Read the model definition and answer for the solid it produces. Units are mm, in the model's axes. A direction names the side the tool comes from. Coordinates: 2 decimals unless noted, no trailing zeros. Order: outer loops, then holes, each group sorted by start corner. A loop starts at its lowest first (then second) coordinate and runs counter-clockwise, first axis right, second up. Notation, with made-up numbers: M 83,-4 L 108,-4 A26 cw 108,28 Z; hole C -29.75,1.25 d9. An arc over 180 degrees is marked long. Put each result on its own line as item: value.
from build123d import *

# Parameters (mm, degrees)
BOSS_EXTRUDE1_DEPTH = 2.7
BOSS_EXTRUDE2_DEPTH = 0.6
FILLET1_R           = 0.5
FILLET2_R           = 2.5
FILLET3_R           = 0.5
FILLET4_R           = 1
SKETCH3_R           = 1
CUT_EXTRUDE1_DEPTH  = 15.611382549


with BuildPart() as part:
    # Sketch1 → Boss-Extrude1 (new body)
    with BuildSketch(Plane.XY):
        with BuildLine():
            Line((-1.082531755, 12.625), (-2.5, 10.169872981))
            Line((-2.5, 10.169872981), (-2.5, 2.449489743))
            ThreePointArc((-2.5, 2.449489743), (-3.463668402, -0.502992247), (-1.7, -3.059411708))
            Line((-1.7, -3.059411708), (-1.7, -7))
            Line((-1.7, -7), (-0.5, -7))
            Line((-0.5, -7), (-0.5, -1.414213562))
            ThreePointArc((-0.5, -1.414213562), (0, 1.5), (0.5, -1.414213562))
            Line((0.5, -1.414213562), (0.5, -7))
            Line((0.5, -7), (1.7, -7))
            Line((1.7, -7), (1.7, -3.059411708))
            ThreePointArc((1.7, -3.059411708), (3.388062941, 0.878082861), (0, 3.5))
            Line((0, 3.5), (0, 9.5))
            Line((0, 9.5), (1.082531755, 11.375))
            ThreePointArc((1.082531755, 11.375), (0.625, 13.082531755), (-1.082531755, 12.625))
        make_face()
    extrude(amount=BOSS_EXTRUDE1_DEPTH)

    # Sketch2 → Boss-Extrude2 (add)
    with BuildSketch(Plane.XY.offset(2.7)):
        with BuildLine():
            Line((0.5, -0.748331477), (0.5, -7))
            Line((0.5, -7), (1.7, -7))
            Line((1.7, -7), (1.7, -3.059411708))
            ThreePointArc((1.7, -3.059411708), (3.388062941, 0.878082861), (0, 3.5))
            Line((0, 3.5), (0, 9.5))
            Line((0, 9.5), (1.082531755, 11.375))
            ThreePointArc((1.082531755, 11.375), (0.625, 13.082531755), (-1.082531755, 12.625))
            Line((-1.082531755, 12.625), (-2.5, 10.169872981))
            Line((-2.5, 10.169872981), (-2.5, 2.449489743))
            ThreePointArc((-2.5, 2.449489743), (-3.463668402, -0.502992247), (-1.7, -3.059411708))
            Line((-1.7, -3.059411708), (-1.7, -7))
            Line((-1.7, -7), (-0.5, -7))
            Line((-0.5, -7), (-0.5, -0.748331477))
            ThreePointArc((-0.5, -0.748331477), (0, 0.9), (0.5, -0.748331477))
        make_face()
    extrude(amount=BOSS_EXTRUDE2_DEPTH)

    # Fillet1
    fillet1_edges = [part.edges().sort_by_distance(p)[0] for p in [
        (-0.5, -0.748331477, 3),
        (0.5, -0.748331477, 3),
    ]]
    fillet(fillet1_edges, radius=FILLET1_R)

    # Fillet2
    fillet2_edges = [part.edges().sort_by_distance(p)[0] for p in [
        (-2.5, 2.449489743, 1.65),
        (-2.5, 10.169872981, 1.65),
        (0, 9.5, 1.65),
        (0, 3.5, 1.65),
    ]]
    fillet(fillet2_edges, radius=FILLET2_R)

    # Fillet3
    fillet3_edges = [part.edges().sort_by_distance(p)[0] for p in [
        (-1.7, -3.059411708, 1.65),
        (1.7, -3.059411708, 1.65),
    ]]
    fillet(fillet3_edges, radius=FILLET3_R)

    # Fillet4
    fillet4_edges = [part.edges().sort_by_distance(p)[0] for p in [
        (-1.1, -7, 0),
        (1.1, -7, 0),
        (1.1, -7, 3.3),
        (-1.1, -7, 3.3),
    ]]
    fillet(fillet4_edges, radius=FILLET4_R)

    # Sketch3 → Cut-Extrude1 (cut, through all)
    with BuildSketch(Plane.ZY.offset(1.7)):
        with Locations((1.65, -5.170329309)):
            Circle(SKETCH3_R)
    extrude(amount=-CUT_EXTRUDE1_DEPTH, mode=Mode.SUBTRACT)


solid = part.part
Q1. Find section A-A on y = 0. Write down the section's boundary in (x, z).
Answers below:
outline: M -3.5,0 L -1.5,0 L -1.5,2.7 L -0.9,2.7 L -0.9,3.3 L -3.5,3.3 Z; M 0.9,2.7 L 1.5,2.7 L 1.5,0 L 3.5,0 L 3.5,3.3 L 0.9,3.3 Z
Q2. For a pull along Y with two mould halves and no side action, classify faces 1 (the face through (-2.4, 10.2, 1.7)), 2 (the face through (1.108, -6.715, 0.301)), 3 (the face through (0.704, 10.718, 1.627)), 4 (the face through (0.5, -4, 2)) as +Y half, -Y half, draft (parallel to the pull), parting line (faces both ways), or undercut.
Answers below:
face 1: +Y half
face 2: -Y half
face 3: undercut
face 4: draft
Q3. Consider line 1 along X through (y, z) = (-3.5, 1.9); line 2 along Y through (x, z) = (0.95, 1.65); line 3 along X through (y, z) = (0, 2.95). Determine where each line is inside the solid, lowest interval first.
Answers below:
line 1: x = -1.7 to -0.5, 0.5 to 1.7
line 2: y = -7 to -6.17, -4.17 to -1.16, 1.16 to 3.49, 11.15 to 12.81
line 3: x = -3.5 to -0.9, 0.9 to 3.5
Q4. Given pin 1 (2 mm diameter, centred on x = 0, y = 0, fed in from -Z), flat-ended and moving along its own axis, determine where the tip first touches the part or whether it passes through.
Answers below:
pin 1: stops at z = 2.7
Q5. Find section C-C on z = 0.2. Write down the section's boundary in (x, y) (3 decimals), plus the area to 3 significant figures.
Answers below:
outline: M -2.917,1.935 A3.5 ccw -1.925,-2.923 A0.5 cw -1.7,-3.341 L -1.7,-6.6 L -0.5,-6.6 L -0.5,-1.414 A1.5 cw long 0.5,-1.414 L 0.5,-6.6 L 1.7,-6.6 L 1.7,-3.341 A0.5 cw 1.925,-2.923 A3.5 ccw 1.458,3.182 A2.5 cw 0,5.454 L 0,8.83 A2.5 cw 0.335,10.08 L 1.083,11.375 A1.25 ccw -1.083,12.625 L -2.165,10.75 A2.5 ccw -2.5,9.5 L -2.5,3.317 A2.5 cw Z
area: 63.4 mm^2
Q6. Find section B-B on z = 1.65. Write down the section's boundary in (x, y) (3 decimals).
Answers below:
outline: M -2.917,1.935 A3.5 ccw -1.925,-2.923 A0.5 cw -1.7,-3.341 L -1.7,-4.17 L -0.5,-4.17 L -0.5,-1.414 A1.5 cw long 0.5,-1.414 L 0.5,-4.17 L 1.7,-4.17 L 1.7,-3.341 A0.5 cw 1.925,-2.923 A3.5 ccw 1.458,3.182 A2.5 cw 0,5.454 L 0,8.83 A2.5 cw 0.335,10.08 L 1.083,11.375 A1.25 ccw -1.083,12.625 L -2.165,10.75 A2.5 ccw -2.5,9.5 L -2.5,3.317 A2.5 cw Z; M -1.7,-7 L -0.5,-7 L -0.5,-6.17 L -1.7,-6.17 Z; M 0.5,-7 L 1.7,-7 L 1.7,-6.17 L 0.5,-6.17 Z
Q7. A tool of negligible diameter and unlimited length cuts with its end or side. For faces 5 (the face through (1.7, -4, 2)), 6 (the face through (-0.06, 1.5, 1.33)), 7 (the face through (0, 7, 2)), from which of +Z, -Z, +X, -X, +Y, -Y can it reach the whole face along a straight path? Write none if from no direction.
Answers below:
face 5: +Z, -Z, +X, -Y
face 6: -Z
face 7: +Z, -Z, +X
Q8. Find section D-D on y = -4.75. Write down the section's boundary in (x, z).
Answers below:
outline: M -1.7,0 L -0.5,0 L -0.5,0.74 L -1.7,0.74 Z; M -1.7,2.56 L -0.5,2.56 L -0.5,3.3 L -1.7,3.3 Z; M 0.5,0 L 1.7,0 L 1.7,0.74 L 0.5,0.74 Z; M 0.5,2.56 L 1.7,2.56 L 1.7,3.3 L 0.5,3.3 Z
